Verification items for the finished model (mm, model axes). Face numbers are marked on the shaded views. A direction names the side the tool comes from. Round coordinates to 2 decimals unless told otherwise and drop trailing zeros. Write each loop counter-clockwise with the first axis right and the second up, starting at its lowest first coordinate (ties: lowest second). Pieces come first, ordered by that corner, then holes. Notation, with made-up numbers: (-27.75, 57) - (-15.75, 57) arc R32 ccw to (-15.75, 95) - close; hole circle Ø10 at (43, 65.5). An arc over 180 degrees is marked (long way). Answer as a JSON object with one key per item and string values.
```python
from build123d import *

# Parameters (mm, degrees)
SKETCH1_W           = 25.4
SKETCH1_H           = 76.2
BOSS_EXTRUDE1_DEPTH = 25.4
SKETCH10_W          = 19.05
SKETCH10_H          = 76.2
CUT_EXTRUDE5_DEPTH  = 19.05
BOSS_EXTRUDE2_START = -6.35
SKETCH12_R          = 3.175
SKETCH12_R_2        = 1.849999983
BOSS_EXTRUDE2_DEPTH = 9.525
BOSS_EXTRUDE3_START = -6.35
SKETCH13_W          = 12.7
SKETCH13_H          = 12.7
BOSS_EXTRUDE3_DEPTH = 12.7
SKETCH14_R          = 3.175
SKETCH14_R_2        = 1.849999983
BOSS_EXTRUDE4_DEPTH = 9.525
SKETCH15_R          = 1.700000029
CUT_EXTRUDE6_DEPTH  = 7.35


with BuildPart() as part:
    # Sketch1 → Boss-Extrude1 (new body)
    with BuildSketch(Plane.XY):
        with Locations((12.7, 38.1)):
            Rectangle(SKETCH1_W, SKETCH1_H)
    extrude(amount=-BOSS_EXTRUDE1_DEPTH)

    # Sketch10 → Cut-Extrude5 (cut)
    with BuildSketch(Plane(origin=(25.4, 0, 0), x_dir=(0, 0, -1), z_dir=(1, 0, 0))):
        with Locations((9.525, 38.1)):
            Rectangle(SKETCH10_W, SKETCH10_H)
    extrude(amount=-CUT_EXTRUDE5_DEPTH, mode=Mode.SUBTRACT)

    # Sketch12 → Boss-Extrude2 (add)
    with BuildSketch(Plane(origin=(0, 0, -25.4), x_dir=(-1, 0, 0), z_dir=(0, 0, -1)).offset(BOSS_EXTRUDE2_START)):
        with Locations((-19.05, 57.15)):
            Circle(SKETCH12_R)
        with Locations((-19.05, 57.15)):
            Circle(SKETCH12_R_2, mode=Mode.SUBTRACT)
    extrude(amount=-BOSS_EXTRUDE2_DEPTH)

    # Sketch13 → Boss-Extrude3 (add)
    with BuildSketch(Plane(origin=(0, 0, -25.4), x_dir=(-1, 0, 0), z_dir=(0, 0, -1)).offset(BOSS_EXTRUDE3_START)):
        with Locations((-19.05, 6.35)):
            Rectangle(SKETCH13_W, SKETCH13_H)
    extrude(amount=-BOSS_EXTRUDE3_DEPTH)

    # Sketch14 → Boss-Extrude4 (add)
    with BuildSketch(Plane.XY.offset(-6.35)):
        with Locations((19.05, 6.35)):
            Circle(SKETCH14_R)
        with Locations((19.05, 6.35)):
            Circle(SKETCH14_R_2, mode=Mode.SUBTRACT)
    extrude(amount=BOSS_EXTRUDE4_DEPTH)

    # Sketch15 → Cut-Extrude6 (cut, through all)
    with BuildSketch(Plane(origin=(6.35, 0, 0), x_dir=(0, 0, -1), z_dir=(1, 0, 0))):
        with Locations((4.7625, 69.85)):
            Circle(SKETCH15_R)
        with Locations((14.2875, 69.85)):
            Circle(SKETCH15_R)
        with Locations((4.7625, 19.05)):
            Circle(SKETCH15_R)
        with Locations((14.2875, 19.05)):
            Circle(SKETCH15_R)
    extrude(amount=-CUT_EXTRUDE6_DEPTH, mode=Mode.SUBTRACT)


solid = part.part
```
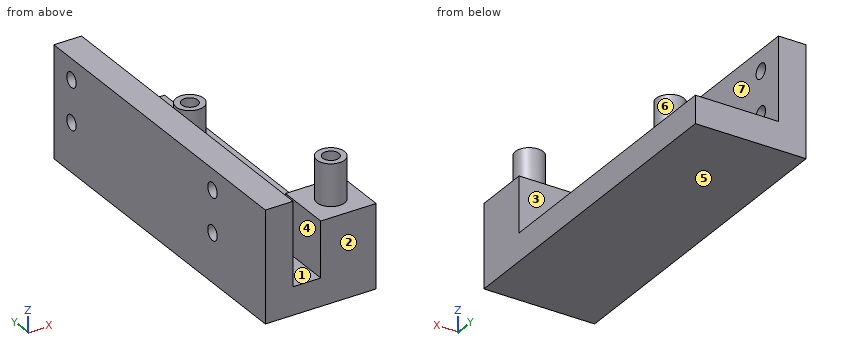
1. Go/stop test with flat-tipped pins: pin 1 (15 mm diameter, centred on x = 20.5, y = 19, fed in from +Z); pin 2 (2.5 mm diameter, centred on y = 69.85, z = -14.29, fed in from +X) (3 decimals); pin 3 (1.9 mm diameter, centred on x = 4.5, y = 46, fed in from +Z); pin 4 (14 mm diameter, centred on x = 20, z = -11.5, fed in from +Y) (3 decimals). Record where each tip stops, or that it passes through.
Completed:
{"pin 1": "stops at z = -6.35", "pin 2": "passes through", "pin 3": "stops at z = 0", "pin 4": "stops at y = 60.325"}
2. Cross-section at B-B (y = 57.15). Record the boundary of the cut face in (x, z) (3 decimals), plus the area to 3 significant figures.
Completed:
{"outline": "(0, -25.4) - (25.4, -25.4) - (25.4, -19.05) - (22.225, -19.05) - (22.225, -9.525) - (20.9, -9.525) - (20.9, -19.05) - (17.2, -19.05) - (17.2, -9.525) - (15.875, -9.525) - (15.875, -19.05) - (6.35, -19.05) - (6.35, 0) - (0, 0) - close", "area": "307 mm^2"}
3. Cross-section at A-A (y = 69.85). Record the boundary of the cut face in (x, z), plus the area to 3 significant figures.
Completed:
{"outline": "(0, -25.4) - (25.4, -25.4) - (25.4, -19.05) - (6.35, -19.05) - (6.35, -15.99) - (0, -15.99) - close; (0, -12.59) - (6.35, -12.59) - (6.35, -6.46) - (0, -6.46) - close; (0, -3.06) - (6.35, -3.06) - (6.35, 0) - (0, 0) - close", "area": "239 mm^2"}
4. Mould release check, pull along Y, two halves, no side actions. Record for the marked faces 1, 2, 3 and 4: released by +Y, released by -Y, zero draft, split by the parting line, or undercut.
Completed:
{"face 1": "undercut", "face 2": "released by -Y", "face 3": "undercut", "face 4": "zero draft"}
5. Cross-section at C-C (z = -4.5). Record the boundary of the cut face in (x, y) (3 decimals), plus the area to 3 significant figures.
Completed:
{"outline": "(0, 0) - (6.35, 0) - (6.35, 17.37) - (0, 17.37) - close; (0, 20.73) - (6.35, 20.73) - (6.35, 68.17) - (0, 68.17) - close; (0, 71.53) - (6.35, 71.53) - (6.35, 76.2) - (0, 76.2) - close; circle Ø6.35 at (19.05, 6.35); hole circle Ø3.7 at (19.05, 6.35)", "area": "462 mm^2"}
6. Access from +Z, -Z, +X, -X, +Y, -Y to the whole of each face (thin tool, end or side, straight path). Record for the marked faces 5, 6 and 7.
Completed:
{"face 5": "-Z, +X, -X, +Y, -Y", "face 6": "+Z", "face 7": "+Z, +Y, -Y"}
7. Cross-section at D-D (x = 19.05). Record the boundary of the cut face in (y, z) (3 decimals).
Completed:
{"outline": "(0, -25.4) - (76.2, -25.4) - (76.2, -19.05) - (60.325, -19.05) - (60.325, -9.525) - (59, -9.525) - (59, -19.05) - (55.3, -19.05) - (55.3, -9.525) - (53.975, -9.525) - (53.975, -19.05) - (12.7, -19.05) - (12.7, -6.35) - (9.525, -6.35) - (9.525, 3.175) - (8.2, 3.175) - (8.2, -6.35) - (4.5, -6.35) - (4.5, 3.175) - (3.175, 3.175) - (3.175, -6.35) - (0, -6.35) - close"}
8. Material ranges on probe 1 along Z at (x, y) = (4.25, 69.85); probe 2 along Y at (x, z) = (19.05, -11.5) (3 decimals); probe 3 along Y at (x, z) = (18.25, -15.25), recorded low to high. Write a range as from..to.
Completed:
{"probe 1": "z = -25.4..-15.99, -12.59..-6.46, -3.06..0", "probe 2": "y = 0..12.7, 53.975..55.3, 59..60.325", "probe 3": "y = 0..12.7, 54.08..55.48, 58.82..60.22"}
